Here's how the part is built. I have some questions about the finished solid (model axes, mm). A direction names the side the tool comes from. Give positions to 0.01 mm unless a question says otherwise; leave off trailing zeros. Write each loop counter-clockwise with the first axis right and the second up, starting at its lowest first coordinate (ties: lowest second). Pieces come first, ordered by that corner, then holes. Notation, with made-up numbers: M 14.25,83 L 49.25,83 A25 ccw 49.25,115 Z; hole C 49,41.25 d1. An arc over 180 degrees is marked long. Answer as CSV lines item,"result". Start each with the question number.
Q1. Thinking about a two-plate mould opening in Z: for faces 4 (the flat face through (68, 25, 30)), 5 (the flat face through (7.4, 32.33, 79.72)), 6 (the flat face through (41, 35, 15)), which applies, +Z half, -Z half, draft (parallel to the pull), parting line (faces both ways), or undercut?
Q2. For pin 1 (4 mm diameter, centred on x = 32.5, y = 38, fed in from +Z); pin 2 (8 mm diameter, centred on y = 24, z = 46.5, fed in from +X); pin 3 (24 mm diameter, centred on x = 71.5, z = 39.5, fed in from -Y), each with a flat end and sliding along its axis, tell me the tip position at first contact or that it passes through.
Q3. If I drill on line 1 along Z through (x, y) = (73.5, 29); line 2 along X through (y, z) = (4.5, 59.5); line 3 along X through (y, z) = (30, 91), over which ranges is the centre line in solid material (lowest first)?
Q4. Suppose I cut it at B-B (x = 59). Write out the boundary of the cut face in (y, z), then the cut area to 3 significant figures.
Q5. Suppose I cut it at C-C (z = 56). Write out the boundary of the cut face in (x, y).
Q6. Suppose I cut it at D-D (y = 42). Write out the boundary of the cut face in (x, z), then the cut area to 3 significant figures.
Q7. On a 3-axis mill with a long thin cutter (end or side, diameter ignored), from which of +Z, -Z, +X, -X, +Y, -Y can I reach the whole of each face in a straight line? I mean faces 1 (the flat face through (52, 20, 49)), 2 (the flat face through (35, 32, 37)), 3 (the flat face through (68, 25, 60)). Say none if no direction works.
```python
from build123d import *

# Parameters (mm, degrees)
F1_DEPTH = 60
F2_DEPTH = 15
F3_DEPTH = 100
F4_DEPTH = 100
F5_W     = 49.251026
F5_H     = 30
F6_DEPTH = 10


with BuildPart() as f1:
    # F0 (on Top) → F1 (new body)
    with BuildSketch(Plane.XY):
        Polygon((0, 45), (0, 20), (15, 45), align=None)
        Polygon((0, 20), (0, 0), (35, 0), (35, 20), (35, 20.001), (35, 45), (15, 45), align=None)
    extrude(amount=F1_DEPTH)

    # F0 (on Top) → F2 (join)
    with BuildSketch(Plane.XY):
        Polygon((35, 45), (35, 20.001), (50, 45), align=None)
    extrude(amount=F2_DEPTH)

    # F0 (on Top) → F3 (join)
    with BuildSketch(Plane.XY):
        Polygon((0, 45), (0, 20), (15, 45), align=None)
    extrude(amount=F3_DEPTH)

    # F0 (on Top) → F4 (join)
    with BuildSketch(Plane.XY):
        Polygon((35, 20.001), (35, 20), (80, 20), (100, 45), (50, 45), align=None)
    extrude(amount=F4_DEPTH)

    # F5 (on face) → F6 (cut)
    with BuildSketch(Plane.XZ.offset(-20)):
        with Locations((79.625513, 45)):
            Rectangle(F5_W, F5_H)
    extrude(amount=-F6_DEPTH, mode=Mode.SUBTRACT)


solid = f1.part
```
Resolved:
1,face 4,"undercut"
1,face 5,"draft"
1,face 6,"+Z half"
2,pin 1,"z = 60"
2,pin 2,"x = 55"
2,pin 3,"y = 20"
3,line 1,"0 to 30, 60 to 100"
3,line 2,"0 to 35"
3,line 3,"0 to 6, 41 to 88"
4,outline,"M 20,0 L 45,0 L 45,100 L 20,100 L 20,60 L 30,60 L 30,30 L 20,30 Z"
4,area,"2,200 mm^2"
5,outline,"M 0,0 L 35,0 L 35,20 L 55,20 L 55,30 L 88,30 L 100,45 L 50,45 L 35,20 L 35,45 L 0,45 Z"
6,outline,"M 0,0 L 97.6,0 L 97.6,100 L 48.2,100 L 48.2,15 L 35,15 L 35,60 L 13.2,60 L 13.2,100 L 0,100 Z"
6,area,"7,770 mm^2"
7,face 1,"+Z, -Z, +X, -Y"
7,face 2,"+Z, +Y"
7,face 3,"+X, -Y"
